Build history of the part. All positions in model axes, mm. A direction names the side the tool comes from. Give positions to 0.01 mm unless a question says otherwise; leave off trailing zeros. Order: outer loops, then holes, each group sorted by start corner. A loop starts at its lowest first (then second) coordinate and runs counter-clockwise, first axis right, second up. Notation, with made-up numbers: (62, 61.25) - (117, 61.25) arc R10 cw to (117, 65.25) - close; hole circle Ø1 at (-20, -5). An arc over 180 degrees is marked (long way). Write each question's results on one line, items separated by ' | '. Start each with the question number.
1) Cut at D-D on z = -45. List the corners of the cut face in (x, y).
2) Tool access for faces 5 (the face through (35, 20, -24)), 6 (the face through (13, 38, -45)), 7 (the face through (2.42, 1.48, -32.18)): list every direction of +Z, -Z, +X, -X, +Y, -Y with a clear straight run to the whole face (end or side of a thin tool).
3) Drop flat-ended pins along their axis: pin 1 Ø6 at (x, y) = (11, 31) entering from -Z; pin 2 Ø3 at (y, z) = (24.5, -10) entering from -X; pin 3 Ø1.5 at (y, z) = (24.5, -32) entering from -X. Give the stop position or say it passes through.
4) Cut at A-A on x = 17. List the corners of the cut face in (y, z).
5) Two-plate mould, pull along Y, no slides. Class faces 1 (the face through (35.72, 9.57, -31.79)), 2 (the face through (19, 0, -18)), 3 (the face through (38, 19, -24)), 4 (the face through (19, 39.5, -18)): +Y half, -Y half, draft (parallel to the pull), parting line (faces both ways), or undercut.
6) Drill centre lines: line 1 along Y through (x, z) = (35.1, -10); line 2 along Z through (x, y) = (30, 38); line 3 along Y through (x, z) = (28, -16.5). Where is each one in solid material? Low to high. Write a range as from..to.
7) Cut at C-C on x = 3.5. List the corners of the cut face in (y, z), plus the area to 3 significant figures.
8) Cut at B-B on z = -4. List the corners of the cut face in (x, y).
Autodesk Inventor part; units mm, degrees
ref_plane "YZ Plane" through (0, 0, 0) normal (1, 0, 0) x (0, 1, 0)
ref_plane "XZ Plane" through (0, 0, 0) normal (0, 1, 0) x (-1, 0, 0)
ref_plane "XY Plane" through (0, 0, 0) normal (0, 0, 1) x (1, 0, 0)
sketch "スケッチ1" plane through (0, 0, 0) normal (0, 1, 0) x (-1, 0, 0)
  line L0 (0, 0) -> (-38, 0)
  line L1 (-38, 0) -> (-38, -48)
  line L2 (-38, -48) -> (0, -48)
  line L3 (0, -48) -> (0, 0)
  dimension "d0" = 48
  dimension "d1" = 38
extrude "押し出し1" add sketch "スケッチ1" along normal blind 39.5
sketch "スケッチ2" plane through (38, 0, -48) normal (0, 0, -1) x (-1, 0, 0)
  line L0 (3, 36.5) -> (59.072, 36.5)
  line L1 (59.072, 36.5) -> (59.072, 3)
  line L2 (59.072, 3) -> (3, 3)
  line L3 (3, 3) -> (3, 36.5)
  line L4 (0, 39.5) -> (38, 39.5)
  line L5 (0, 0) -> (38, 0)
  line L6 (0, 0) -> (0, 39.5)
  dimension "d4" = 33.5
  dimension "d6" = 3
  dimension "d7" = 3
extrude "押し出し2" cut sketch "スケッチ2" against normal blind 100
sketch "スケッチ3" plane through (0, 39.5, 0) normal (0, 1, 0) x (1, 0, 0)
  line L0 (38, 48) -> (0, 48)
  line L1 (38, 0) -> (38, 48)
  point P0 (0, 0)
  point P1 (17, 32)
  dimension "d10" = 16
  dimension "d11" = 21
hole "穴1" at (17, 39.5, -32) direction (0, -1, 0) diameter 22 end through all
sketch "スケッチ4" plane through (0, 39.5, 0) normal (0, 1, 0) x (1, 0, 0)
  line L0 (0, 0) -> (38, 0)
  line L1 (38, 0) -> (38, 48)
  point P0 (30.5, 4)
  point P1 (30.5, 31)
  point P2 (3.5, 4)
  point P3 (3.5, 31)
  point P4 (3.5, 4)
  dimension "d19" = 4
  dimension "d20" = 7.5
  dimension "d23" = 27
  dimension "d26" = 27
hole "穴2" at (30.5, 39.5, -4) at (30.5, 39.5, -31) at (3.5, 39.5, -31) at (3.5, 39.5, -4) direction (0, -1, 0) diameter 3.2 end through all
sketch "スケッチ6" plane through (38, 0, 0) normal (1, 0, 0) x (0, 0, -1)
  line L0 (0, 39.5) -> (48, 39.5)
  line L1 (0, 0) -> (0, 39.5)
  point P0 (10, 24.5)
  point P1 (32, 24.5)
  point P2 (10, 9.5)
  point P3 (32, 9.5)
  dimension "d45" = 15
  dimension "d46" = 10
  dimension "d49" = 22
  dimension "d52" = 15
fillet "フィレット1" radius 2 2 edges at (35, 3, -24) (35, 36.5, -24)
sketch "スケッチ7" plane through (0, 39.5, 0) normal (0, 1, 0) x (1, 0, 0)
  line L0 (38, 48) -> (0, 48)
  line L1 (13, 48) -> (21, 48)
  line L2 (21, 48) -> (21, 39.3329)
  line L3 (21, 39.3329) -> (13, 39.3329)
  line L4 (13, 39.3329) -> (13, 48)
  circle A0 centre (17, 32) radius 11
  point P0 (0, 0)
  point P1 (13, 42.247)
  point P2 (21, 42.247)
  dimension "d69" = 8
  dimension "d70" = 4
extrude "押し出し3" cut sketch "スケッチ7" against normal blind 3 contours L2 A0 L4 L0
sketch "スケッチ8" plane through (35, 5, -48) normal (-1, 0, 0) x (0, 0, 1)
  line L0 (16, 4.5) -> (38, 4.5)
  line L1 (38, 4.5) -> (38, 19.5)
  line L2 (38, 19.5) -> (16, 19.5)
  line L3 (16, 19.5) -> (16, 4.5)
  line L4 (48, 34.5) -> (48, 0)
  line L5 (48, 34.5) -> (0, 34.5)
  point P0 (48, -5)
  point P1 (48, 29.5)
  dimension "d73" = 10
  dimension "d74" = 22
  dimension "d75" = 15
  dimension "d76" = 15
hole "穴5" at (35, 9.5, -10) at (35, 9.5, -32) at (35, 24.5, -32) at (35, 24.5, -10) direction (1, 0, 0) diameter 2.5 depth 0.1 tip angle 118
properties part number "サーボモータ固定用２軸目3mm改_printer"
Results:
1) outline: (0, 0) - (38, 0) - (38, 39.5) - (21, 39.5) - (21, 36.5) - (33, 36.5) arc R2 cw to (35, 34.5) - (35, 5) arc R2 cw to (33, 3) - (0, 3) - close; (0, 36.5) - (13, 36.5) - (13, 39.5) - (0, 39.5) - close
2) face 5: +Z, -Z, -X | face 6: -Z, +Y | face 7: +Y, -Y
3) pin 1: through | pin 2: x = 35 | pin 3: x = 35.4
4) outline: (0, -48) - (3, -48) - (3, -43) - (0, -43) - close; (0, -21) - (3, -21) - (3, 0) - (0, 0) - close; (36.5, -21) - (39.5, -21) - (39.5, 0) - (36.5, 0) - close
5) face 1: undercut | face 2: -Y half | face 3: draft | face 4: +Y half
6) line 1: 0..8.25, 10.75..23.25, 25.75..39.5 | line 2: -48..-32.52, -29.48..-5.52, -2.48..0 | line 3: 0..3, 36.5..39.5
7) outline: (0, -48) - (3, -48) - (3, -32.6) - (0, -32.6) - close; (0, -29.4) - (3, -29.4) - (3, -5.6) - (0, -5.6) - close; (0, -2.4) - (3, -2.4) - (3, 0) - (0, 0) - close; (36.5, -48) - (39.5, -48) - (39.5, -32.6) - (36.5, -32.6) - close; (36.5, -29.4) - (39.5, -29.4) - (39.5, -5.6) - (36.5, -5.6) - close; (36.5, -2.4) - (39.5, -2.4) - (39.5, 0) - (36.5, 0) - close | area: 250 mm^2
8) outline: (0, 0) - (1.9, 0) - (1.9, 3) - (0, 3) - close; (0, 36.5) - (1.9, 36.5) - (1.9, 39.5) - (0, 39.5) - close; (5.1, 0) - (28.9, 0) - (28.9, 3) - (5.1, 3) - close; (5.1, 36.5) - (28.9, 36.5) - (28.9, 39.5) - (5.1, 39.5) - close; (32.1, 0) - (38, 0) - (38, 39.5) - (32.1, 39.5) - (32.1, 36.5) - (33, 36.5) arc R2 cw to (35, 34.5) - (35, 5) arc R2 cw to (33, 3) - (32.1, 3) - close
